```python
from build123d import *

# Parameters (mm, degrees)
F0_W     = 41
F0_H     = 41
F0_R     = 1
F0_R_2   = 11
F0_R_3   = 2.5
F1_DEPTH = 37
F2_SIZE  = 5
F3_DEPTH = 2
F4_DEPTH = 10


with BuildPart() as f1:
    # F0 (on Top) → F1 (new body)
    with BuildSketch(Plane.XY):
        with Locations((-20.5, 20.5)):
            Rectangle(F0_W, F0_H)
        with Locations((-36, 5)):
            Circle(F0_R, mode=Mode.SUBTRACT)
        with Locations((-5, 5)):
            Circle(F0_R, mode=Mode.SUBTRACT)
        with Locations((-36, 36)):
            Circle(F0_R, mode=Mode.SUBTRACT)
        with Locations((-20.5, 20.5)):
            Circle(F0_R_2, mode=Mode.SUBTRACT)
        with Locations((-5, 36)):
            Circle(F0_R, mode=Mode.SUBTRACT)
        with Locations((-20.5, 20.5)):
            Circle(F0_R_2)
        with Locations((-20.5, 20.5)):
            Circle(F0_R_3, mode=Mode.SUBTRACT)
    extrude(amount=F1_DEPTH)

    # F2
    f2_edges = [f1.edges().sort_by_distance(p)[0] for p in [
        (0, 41, 18.5),
        (-41, 41, 18.5),
        (0, 0, 18.5),
        (-41, 0, 18.5),
    ]]
    chamfer(f2_edges, length=F2_SIZE)

    # F0 (on Top) → F3 (join)
    with BuildSketch(Plane.XY):
        with Locations((-20.5, 20.5)):
            Circle(F0_R_2)
        with Locations((-20.5, 20.5)):
            Circle(F0_R_3, mode=Mode.SUBTRACT)
    extrude(amount=-F3_DEPTH)

    # F0 (on Top) → F4 (join)
    with BuildSketch(Plane.XY):
        with Locations((-20.5, 20.5)):
            Circle(F0_R_3)
    extrude(amount=-F4_DEPTH)


solid = f1.part
```
Check sheet for the modelled part. Datum: model origin and axes. Units: mm. A direction names the side the tool comes from. Coordinates: 2 decimals unless noted, no trailing zeros. Order: outer loops, then holes, each group sorted by start corner. A loop starts at its lowest first (then second) coordinate and runs counter-clockwise, first axis right, second up. Notation, with made-up numbers: M 84,11.5 L 114,11.5 A8 cw 114,22.5 Z; hole C 45.5,35 d1. An arc over 180 degrees is marked long. One line per question, with ' | ' between items. Start each with the question number.
Item 1: Material ranges on line 1 (Y direction, x = -5, z = 18); line 2 (Z direction, x = -14, y = 35.5); line 3 (X direction, y = 5.5, z = 25), recorded low to high.
Item 2: Mould release check, pull along Y, two halves, no side actions. Record for faces 1 (the flat face through (-18, 18, -2)), 2 (the flat face through (-21, 0, 18)), 3 (the cylindrical face through (-5, 6, 18)): pulls with the +Y half, pulls with the -Y half, needs draft (parallel to the pull), parting line crosses it, or undercut.
Item 3: Sectioned sample at A-A on z = 4. Record the cut outline in (x, y), and give its area (3 significant figures).
Item 4: Gauge pin test, flat ends, axial feed: P1, Ø6.5, axis at x = -17.5, y = 15.5, coming from the -Z side; P2, Ø1.5, axis at x = -20, y = 21, coming from the +Z side; P3, Ø2.5, axis at x = -5, y = 5, coming from the -Z side. Record the tip position at first contact, or that the pin passes through.
Item 5: Sectioned sample at D-D on x = -15. Record the cut outline in (y, z), and give its area (3 significant figures).
Item 6: Access from +Z, -Z, +X, -X, +Y, -Y to the whole of each face (thin tool, end or side, straight path). Record for faces 4 (the cylindrical face through (-22.34, 22.19, 18.24)), 5 (the flat face through (-12, 12, 0)), 6 (the flat face through (-2, 3, 18)).
Item 7: Sectioned sample at C-C on y = 21.5. Record the cut outline in (x, z).
Item 8: Sectioned sample at B-B on x = -20.5. Record the cut outline in (y, z), and give its area (3 significant figures).
Answer below:
1) line 1: y = 0 to 4, 6 to 35, 37 to 41 | line 2: z = 0 to 37 | line 3: x = -41 to -36.87, -35.13 to -5.87, -4.13 to 0
2) face 1: needs draft | face 2: pulls with the -Y half | face 3: undercut
3) outline: M -41,5 L -36,0 L -5,0 L 0,5 L 0,36 L -5,41 L -36,41 L -41,36 Z; hole C -36,5 d2; hole C -36,36 d2; hole C -20.5,20.5 d5; hole C -5,5 d2; hole C -5,36 d2 | area: 1,600 mm^2
4) P1: stops at z = -2 | P2: stops at z = 0 | P3: stops at z = 0
5) outline: M 0,0 L 10.97,0 L 10.97,-2 L 30.03,-2 L 30.03,0 L 41,0 L 41,37 L 0,37 Z | area: 1,560 mm^2
6) face 4: +Z | face 5: -Z | face 6: +Z, -Z, +X, -Y
7) outline: M -41,0 L -31.45,0 L -31.45,-2 L -22.79,-2 L -22.79,-10 L -18.21,-10 L -18.21,-2 L -9.55,-2 L -9.55,0 L 0,0 L 0,37 L -18.21,37 L -18.21,0 L -22.79,0 L -22.79,37 L -41,37 Z
8) outline: M 0,0 L 9.5,0 L 9.5,-2 L 18,-2 L 18,-10 L 23,-10 L 23,-2 L 31.5,-2 L 31.5,0 L 41,0 L 41,37 L 23,37 L 23,0 L 18,0 L 18,37 L 0,37 Z | area: 1,420 mm^2
